Autodesk Inventor part; units mm, degrees
ref_plane "YZ Plane" through (0, 0, 0) normal (1, 0, 0) x (0, 1, 0)
ref_plane "XY Plane" through (0, 0, 0) normal (0, 0, 1) x (1, 0, 0)
sketch "Sketch1" plane through (0, 0, 0) normal (0, 0, 1) x (1, 0, 0)
  line L0 (0, 0) -> (280, 0)
  line L1 (280, 0) -> (280, 6)
  line L2 (0, 0) -> (0, 6)
  line L3 (0, 6) -> (40, 6)
  line L4 (40, 6) -> (40, 8)
  line L5 (40, 8) -> (278, 8)
  line L6 (278, 8) -> (280, 6)
  point P0 (280, 8)
  dimension "d0" = 280
  dimension "d1" = 8
  dimension "d2" = 6
  dimension "d3" = 40
  dimension "d4" = 2
  dimension "d5" = 2
  dimension "d6" = 45
revolve "Revolution1" add sketch "Sketch1" angle 360 about axis through (0, 0, 0) along (1, 0, 0)
thread "Thread1"
ref_plane "Work Plane1" through (0, 8, 0) normal (0, 1, 0) x (-1, 0, 0)
sketch "Sketch2" plane through (0, 8, 0) normal (0, 1, 0) x (-1, 0, 0)
  circle A0 centre (-270, 0) radius 2.5
  line L0 (-280, 6) -> (-280, -6)
  point P0 (0, 0)
  dimension "d12" = 5
  dimension "d13" = 10
  dimension "d14" = 270
extrude "Extrusion1" cut sketch "Sketch2" against normal through all
Can you work these out from the model? Positions are in its coordinate system, mm. A direction names the side the tool comes from. Round coordinates to 2 decimals unless told otherwise and drop trailing zeros. Loops run counter-clockwise (first coordinate to the right, second up) from the corner with the lowest first, then second, coordinate; pieces in that order, holes last.
Item 1: Suppose I cut it at C-C, the plane x = 229.5. Write out the boundary of the cut face in (y, z), then the cut area to 3 significant figures.
Item 2: Suppose I cut it at B-B, the plane y = 0. Write out the boundary of the cut face in (x, z), then the cut area to 3 significant figures.
Item 3: Please list where these lines run through material, in increasing order: L1, parallel to X at y = -1.5, z = 0; L2, parallel to Z at x = 270, y = 0; L3, parallel to X at y = -5.5, z = -0.5.
Item 4: Suppose I cut it at A-A, the plane z = 0. Write out the boundary of the cut face in (x, y).
Item 5: Which directions (+Z, -Z, +X, -X, +Y, -Y) give clear straight access to the entire face, cutting with the end or side of a thin tool? Please do faces 4 (the flat face through (40, -2, 6)), 5 (the flat face through (280, 0, 0)).
Item 6: If we mould it in two halves opening along X, with no side actions, what happens to faces 1 (the flat face through (0, 0, 0)), 2 (the cylindrical face through (267.69, 0.11, -0.96)), 3 (the cylindrical face through (20, -6, 0))? For each: +X half, -X half, draft (parallel to the pull), parting line (faces both ways), or undercut.
Item 7: Will these pins go through, and if not, where does the flat tip stop? pin 1 Ø2 at (x, y) = (139, -3.5) entering from -Z; pin 2 Ø4 at (x, y) = (70, -5) entering from -Z; pin 3 Ø4 at (x, y) = (168.5, 5) entering from +Z.
Reported:
1. outline: circle Ø16 at (0, 0)
1. area: 201 mm2
2. outline: (0, -6) - (40, -6) - (40, -8) - (278, -8) - (280, -6) - (280, 6) - (278, 8) - (40, 8) - (40, 6) - (0, 6) - close; hole circle Ø5 at (270, 0)
2. area: 4,300 mm2
3. L1: x = 0 to 267.5, 272.5 to 280
3. L2: z = -8 to -2.5, 2.5 to 8
3. L3: x = 0 to 267.55, 272.45 to 280
4. outline: (0, -6) - (40, -6) - (40, -8) - (267.5, -8) - (267.5, 8) - (40, 8) - (40, 6) - (0, 6) - close; (272.5, -8) - (278, -8) - (280, -6) - (280, 6) - (278, 8) - (272.5, 8) - close
5. face 4: -X
5. face 5: +Z, -Z, +X, +Y, -Y
6. face 1: -X half
6. face 2: undercut
6. face 3: draft
7. pin 1: stops at z = -7.6
7. pin 2: stops at z = -7.42
7. pin 3: stops at z = 7.42
